```python
from build123d import *

# Parameters (mm, degrees)
F0_R     = 9
F1_DEPTH = 120
F2_R     = 6.5
F3_DEPTH = 60
F4_R     = 4
F5_DEPTH = 30
F6_R     = 5


with BuildPart() as f1:
    # F0 (on Top) → F1 (new body)
    with BuildSketch(Plane.XY):
        Circle(F0_R)
    extrude(amount=F1_DEPTH)

    # F2 (on face) → F3 (cut)
    with BuildSketch(Plane(origin=(0, 0, 0), x_dir=(1, 0, 0), z_dir=(0, 0, -1))):
        Circle(F2_R)
    extrude(amount=-F3_DEPTH, mode=Mode.SUBTRACT)

    # F4 (on face) → F5 (cut)
    with BuildSketch(Plane(origin=(0, 0, 60), x_dir=(1, 0, 0), z_dir=(0, 0, -1))):
        Circle(F4_R)
    extrude(amount=-F5_DEPTH, mode=Mode.SUBTRACT)

    # F6
    f6_edges = [f1.edges().sort_by_distance(p)[0] for p in [
        (-9, 0, 120),
    ]]
    fillet(f6_edges, radius=F6_R)


solid = f1.part
```
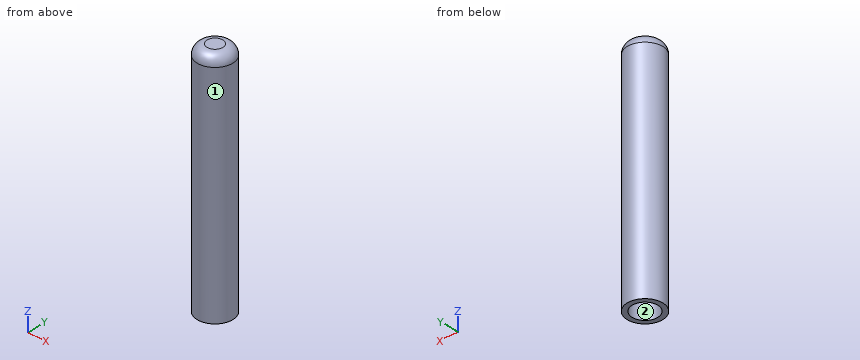
The model under review builds one solid part; all positions refer to its coordinate system, in mm. Face numbers are marked on the shaded views. Round coordinates to 2 decimals unless told otherwise and drop trailing zeros. Loops run counter-clockwise (first coordinate to the right, second up) from the corner with the lowest first, then second, coordinate; pieces in that order, holes last. Notation, with made-up numbers: (30, 27) -> (46, 27) arc R30 ccw to (46, 63) -> close; hole circle Ø6 at (-7.75, 33). An arc over 180 degrees is marked (long way). Answer as a JSON object with one key per item and string values. Group by question number.
1) Mouldability with a two-part tool opening along Y and no side actions: class the marked faces 1 and 2 as released by +Y, released by -Y, zero draft, split by the parting line, or undercut.
2) We need section A-A on z = 11.5. Write out the cut boundary in (x, y).
3) For line 1 (Y direction, x = 0, z = 80); line 2 (Y direction, x = 0, z = 45); line 3 (X direction, y = -0.5, z = 106), list the stretches that pass through material, from the lowest coordinate up. Write a range as [from, to].
4) For pin 1 Ø3 at (y, z) = (-7, 85.5) entering from +X; pin 2 Ø4 at (x, y) = (2.5, -1) entering from -Z; pin 3 Ø2 at (x, z) = (4.5, 57) entering from -Y, all flat-tipped, find the tip position at first contact; note any pin that passes through.
Result set:
{
 "1": {"face 1": "split by the parting line", "face 2": "undercut"},
 "2": {"outline": "circle Ø18 at (0, 0); hole circle Ø13 at (0, 0)"},
 "3": {"line 1": "[-9, -4], [4, 9]", "line 2": "[-9, -6.5], [6.5, 9]", "line 3": "[-8.99, 8.99]"},
 "4": {"pin 1": "x = 7.12", "pin 2": "z = 60", "pin 3": "y = -8.29"}
}
